from build123d import *

# Parameters (mm, degrees)
F0_W     = 30
F0_H     = 70
F1_DEPTH = 3
F2_W     = 30
F2_H     = 3
F3_DEPTH = 20
F4_R     = 2.75
F5_DEPTH = 3.001
F6_R     = 1.75
F7_DEPTH = 23.001


with BuildPart() as f1:
    # F0 (on Front) → F1 (new body)
    with BuildSketch(Plane.XZ):
        with Locations((2.5, 35)):
            Rectangle(F0_W, F0_H)
    extrude(amount=F1_DEPTH)

    # F2 (on face) → F3 (join)
    with BuildSketch(Plane(origin=(0, 0, 0), x_dir=(-1, 0, 0), z_dir=(0, 1, 0))):
        with Locations((-2.5, 1.5)):
            Rectangle(F2_W, F2_H)
    extrude(amount=F3_DEPTH)

    # F4 (on face) → F5 (cut, through all)
    with BuildSketch(Plane.XY.offset(3)):
        with Locations((12.5, 9.75894)):
            Circle(F4_R)
        with Locations((-7.5, 9.75894)):
            Circle(F4_R)
    extrude(amount=-F5_DEPTH, mode=Mode.SUBTRACT)

    # F6 (on face) → F7 (cut, through all)
    with BuildSketch(Plane.XZ.offset(3)):
        with Locations((-9, 65)):
            Circle(F6_R)
        with Locations((-9, 48)):
            Circle(F6_R)
        with Locations((14, 65)):
            Circle(F6_R)
        with Locations((14, 48)):
            Circle(F6_R)
    extrude(amount=-F7_DEPTH, mode=Mode.SUBTRACT)


solid = f1.part
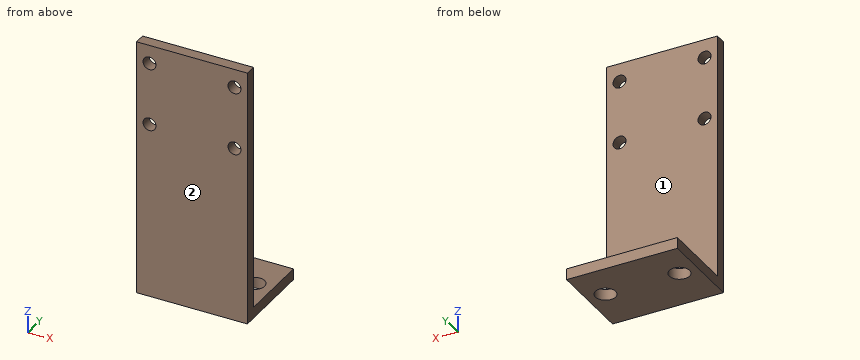
Can you work these out from the model? Positions are in its coordinate system, mm. Face numbers are marked on the shaded views. A direction names the side the tool comes from. Give positions to 0.01 mm unless a question says otherwise; leave off trailing zeros. Order: outer loops, then holes, each group sorted by start corner. A loop starts at its lowest first (then second) coordinate and runs counter-clockwise, first axis right, second up. Notation, with made-up numbers: M -32.75,-12 L -13.75,-12 A32 cw -13.75,17 Z; hole C 56.25,-11 d9. An arc over 180 degrees is marked long. Use a Markdown table: item, result. Add a question column.
Item 1: For the marked faces 1 and 2, which set-ups out of +Z, -Z, +X, -X, +Y, -Y let a thin tool reach every point of the face, with its end or its side?
Item 2: Suppose I cut it at C-C (x = -9). List the corners of the cut face in (y, z) for me.
Item 3: Will these pins go through, and if not, where does the flat tip stop? pin 1 (2 mm diameter, centred on x = -4.5, z = 23.5, fed in from +Y); pin 2 (12 mm diameter, centred on x = -1.5, y = 2, fed in from +Z); pin 3 (2 mm diameter, centred on x = -9, z = 65, fed in from -Y) (1 decimal); pin 4 (6 mm diameter, centred on x = -7.5, y = 8.5, fed in from +Z).
Item 4: Suppose I cut it at D-D (x = 3). List the corners of the cut face in (y, z) for me.
Item 5: If I drill on L1, parallel to Z at x = -9, y = -2.3; L2, parallel to X at y = -1.75, z = 65; L3, parallel to Z at x = -3.5, y = 9.5, over which ranges is the centre line in solid material (lowest first)? Write a range as [from, to].
Item 6: Suppose I cut it at A-A (z = 48). List the corners of the cut face in (x, y) for me, then the cut area to 3 significant figures.
Item 7: Suppose I cut it at B-B (y = 8.25). List the corners of the cut face in (x, z) for me.
Answer sheet:
| question | item | result |
|---|---|---|
| 1 | face 1 | +Z, +X, -X, +Y |
| 1 | face 2 | +Z, -Z, +X, -X, -Y |
| 2 | outline | M -3,0 L 7.45,0 L 7.45,3 L 0,3 L 0,46.25 L -3,46.25 Z; M -3,49.75 L 0,49.75 L 0,63.25 L -3,63.25 Z; M -3,66.75 L 0,66.75 L 0,70 L -3,70 Z; M 12.06,0 L 20,0 L 20,3 L 12.06,3 Z |
| 3 | pin 1 | stops at y = 0 |
| 3 | pin 2 | stops at z = 70 |
| 3 | pin 3 | passes through |
| 3 | pin 4 | stops at z = 3 |
| 4 | outline | M -3,0 L 20,0 L 20,3 L 0,3 L 0,70 L -3,70 Z |
| 5 | L1 | z = [0, 46.25], [49.75, 63.25], [66.75, 70] |
| 5 | L2 | x = [-12.5, -10.75], [-7.25, 12.25], [15.75, 17.5] |
| 5 | L3 | z = [0, 3] |
| 6 | outline | M -12.5,-3 L -10.75,-3 L -10.75,0 L -12.5,0 Z; M -7.25,-3 L 12.25,-3 L 12.25,0 L -7.25,0 Z; M 15.75,-3 L 17.5,-3 L 17.5,0 L 15.75,0 Z |
| 6 | area | 69.0 mm² |
| 7 | outline | M -12.5,0 L -9.8,0 L -9.8,3 L -12.5,3 Z; M -5.2,0 L 10.2,0 L 10.2,3 L -5.2,3 Z; M 14.8,0 L 17.5,0 L 17.5,3 L 14.8,3 Z |
